The listing builds one solid part. Answer for the finished solid, in the listing's coordinates (mm). Coordinates: 2 decimals unless noted, no trailing zeros. Order: outer loops, then holes, each group sorted by start corner. A loop starts at its lowest first (then second) coordinate and runs counter-clockwise, first axis right, second up. Notation, with made-up numbers: (18.5, 41.25) - (47.5, 41.25) arc R16 ccw to (47.5, 66.25) - close; hole circle Ø7 at (52, -29). An arc over 180 degrees is marked (long way). Use one line per item in the form item = value. Start each with the question number.
Item 1: Section A-A, the plane x = -32.5 is taken. Write down the section's boundary in (y, z).
Item 2: The mould has two halves that part along Y. Classify faces 1 (the flat face through (-0.853, 2.778, 12.148)), 2 (the flat face through (-0.85, 48.67, 24.44)), 3 (the flat face through (1, 50.8, 14)), 4 (the flat face through (-0.85, 26.38, 17.14)): released by +Y, released by -Y, zero draft, split by the parting line, or undercut.
Item 3: This flat-tipped pin is pushed along its axis until it touches: pin 1 Ø5 at (x, y) = (-12, 26) entering from +Z. Where does it stop, or does it pass through?
Item 4: Section C-C, the plane z = 19.75 is taken. Write down the section's boundary in (x, y), and give its area (3 significant figures).
Item 5: Section B-B, the plane y = 39.5 is taken. Write down the section's boundary in (x, z).
Item 6: Consider line 1 along X through (y, z) = (25, 17); line 2 along X through (y, z) = (48.5, 7.75); line 3 along Z through (x, y) = (4, 48). Determine where each line is inside the solid, lowest interval first. Write a range as [from, to].
from build123d import *

# Parameters (mm, degrees)
BOSS_EXTRUDE1_DEPTH = 63.5
SKETCH2_W           = 121.92
SKETCH2_H           = 47.512029965
CUT_EXTRUDE1_DEPTH  = 2.54
FILLET1_R           = 2.54


with BuildPart() as part:
    # Sketch1 → Boss-Extrude1 (new body, symmetric)
    with BuildSketch(Plane(origin=(0, 0, 0), x_dir=(0, 0, -1), z_dir=(1, 0, 0))):
        Polygon((0, 0), (0, 50.8), (-26.311818976, 50.8), (-12.7, 0), align=None)
    extrude(amount=BOSS_EXTRUDE1_DEPTH, both=True)

    # Sketch2 → Cut-Extrude1 (cut)
    with BuildSketch(Plane(origin=(0, -3.175, 11.849261314), x_dir=(1, 0, 0), z_dir=(0, -0.258819045, 0.965925826))):
        with Locations((0, 29.583016856)):
            Rectangle(SKETCH2_W, SKETCH2_H)
    extrude(amount=-CUT_EXTRUDE1_DEPTH, mode=Mode.SUBTRACT)

    # Fillet1
    fillet1_edges = [part.edges().sort_by_distance(p)[0] for p in [
        (63.5, 50.8, 13.155909488),
        (-63.5, 50.8, 13.155909488),
        (-63.5, 25.4, 0),
        (0, 50.8, 0),
        (63.5, 25.4, 0),
    ]]
    fillet(fillet1_edges, radius=FILLET1_R)


solid = part.part
Response:
q1.outline = (0, 0) - (48.26, 0) arc R2.54 ccw to (50.8, 2.54) - (50.8, 26.31) - (48.35, 25.65) - (49, 23.2) - (3.11, 10.9) - (2.45, 13.36) - (0, 12.7) - close
q2.face_1 = undercut
q2.face_2 = released by -Y
q2.face_3 = released by +Y
q2.face_4 = undercut
q3.pin_1 = 17.71
q4.outline = (-63.5, 26.31) - (-60.96, 26.31) - (-60.96, 36.12) - (60.96, 36.12) - (60.96, 26.31) - (63.5, 26.31) - (63.5, 48.26) arc R2.54 ccw to (60.96, 50.8) - (-60.96, 50.8) arc R2.54 ccw to (-63.5, 48.26) - close
q4.area = 1,910 mm2
q5.outline = (-63.5, 2.54) arc R2.54 ccw to (-60.96, 0) - (60.96, 0) arc R2.54 ccw to (63.5, 2.54) - (63.5, 23.28) - (60.96, 23.28) - (60.96, 20.65) - (-60.96, 20.65) - (-60.96, 23.28) - (-63.5, 23.28) - close
q6.line_1 = [-63.5, -60.96], [60.96, 63.5]
q6.line_2 = [-63.49, 63.49]
q6.line_3 = [0, 22.93]
